Can you work these out from the model? Positions are in its coordinate system, mm. A direction names the side the tool comes from. Round coordinates to 2 decimals unless told otherwise and drop trailing zeros. Write each loop counter-clockwise with the first axis right and the second up, starting at its lowest first coordinate (ties: lowest second). Pieces come first, ordered by that corner, then holes. Notation, with made-up numbers: (88.5, -26) - (124.5, -26) arc R19 ccw to (124.5, 10) - close; hole circle Ø6 at (-28, 69.25). An arc over 180 degrees is marked (long way). One line per item, written item: value. Start each with the question number.
(1) On a 3-axis mill with a long thin cutter (end or side, diameter ignored), from which of +Z, -Z, +X, -X, +Y, -Y can I reach the whole of each face in a straight line? I mean faces 1 (the face through (-34, 685.8, -14)), 2 (the face through (-31.75, -10, 3)). Say none if no direction works.
(2) I want a section at B-B on x = 4.5. List the corners of the cut face in (y, z) for me, plus the area to 3 significant figures.
(3) If I drill on L1, parallel to X at y = -186, z = 32.5; L2, parallel to Z at x = -34, y = 654.05, over which ranges is the centre line in solid material (lowest first)? Write a range as from..to.
(4) I'm going to push flat-ended pins straight in: pin 1 Ø4 at (x, z) = (-28, 26) entering from +Y; pin 2 Ø18 at (x, y) = (-11.5, 132.5) entering from +Z; pin 3 Ø2 at (y, z) = (-139, 11.5) entering from +X. Where does each tip first touch, or does it pass through?
(5) I want a section at A-A on y = -25.5. List the corners of the cut face in (x, z) for me, plus the area to 3 significant figures.
from build123d import *

# Parameters (mm, degrees)
F1_DEPTH = 685.8
F2_R     = 5.08
F3_R     = 7.14375
F4_DEPTH = 25.4


with BuildPart() as f1:
    # F0 (on Front) → F1 (new body, symmetric)
    with BuildSketch(Plane.XZ):
        Polygon((-31.75, -31.75), (-31.75, 38.1), (-38.1, 38.1), (-38.1, -38.1), (38.1, -38.1), (38.1, -31.75), align=None)
    extrude(amount=F1_DEPTH, both=True)

    # F2
    f2_edges = [f1.edges().sort_by_distance(p)[0] for p in [
        (-31.75, 0, -31.75),
        (-31.75, 0, 38.1),
        (38.1, 0, -31.75),
    ]]
    fillet(f2_edges, radius=F2_R)

    # F3 (on face) → F4 (cut)
    with BuildSketch(Plane(origin=(-38.1, 0, 0), x_dir=(0, -1, 0), z_dir=(-1, 0, 0))):
        with Locations((660.4, 0)):
            Circle(F3_R)
        with Locations((-654.05, 6.35)):
            Circle(F3_R)
    extrude(amount=-F4_DEPTH, mode=Mode.SUBTRACT)


solid = f1.part
Established:
1. face 1: +Z, -Z, +X, -X, +Y
1. face 2: +Z, +X, +Y, -Y
2. outline: (-685.8, -38.1) - (685.8, -38.1) - (685.8, -31.75) - (-685.8, -31.75) - close
2. area: 8,710 mm2
3. L1: -38.1..-31.75
3. L2: -38.1..-0.79, 13.49..37.24
4. pin 1: through
4. pin 2: z = -31.75
4. pin 3: x = -31.75
5. outline: (-38.1, -38.1) - (38.1, -38.1) - (38.1, -36.83) arc R5.08 ccw to (33.02, -31.75) - (-26.67, -31.75) arc R5.08 cw to (-31.75, -26.67) - (-31.75, 33.02) arc R5.08 ccw to (-36.83, 38.1) - (-38.1, 38.1) - close
5. area: 922 mm2
